For this review, take the finished solid that the model builds, in its own axes (mm). A direction names the side the tool comes from. Round coordinates to 2 decimals unless told otherwise and drop trailing zeros. Write each loop counter-clockwise with the first axis right and the second up, starting at its lowest first coordinate (ties: lowest second). Pieces come first, ordered by that corner, then holes.
from build123d import *

# Parameters (mm, degrees)
F0_W     = 20
F0_H     = 23
F0_R     = 2
F1_DEPTH = 3
F2_W     = 20
F2_H     = 3
F3_DEPTH = 20
F4_R     = 2
F5_DEPTH = 3.001
F7_DEPTH = 2
F9_DEPTH = 2
F10_SIZE = 1


with BuildPart() as f1:
    # F0 (on Top) → F1 (new body)
    with BuildSketch(Plane.XY):
        with Locations((10, -11.5)):
            Rectangle(F0_W, F0_H)
        with Locations((10, -13)):
            Circle(F0_R, mode=Mode.SUBTRACT)
    extrude(amount=F1_DEPTH)

    # F2 (on face) → F3 (join)
    with BuildSketch(Plane.XY.offset(3)):
        with Locations((10, -1.5)):
            Rectangle(F2_W, F2_H)
    extrude(amount=F3_DEPTH)

    # F4 (on face) → F5 (cut, through all)
    with BuildSketch(Plane.XZ.offset(3)):
        with Locations((10, 13)):
            Circle(F4_R)
    extrude(amount=-F5_DEPTH, mode=Mode.SUBTRACT)

    # F6 (on face) → F7 (join)
    with BuildSketch(Plane.YZ.offset(20)):
        Polygon((-3, 3), (-3, 23), (-23, 3), align=None)
    extrude(amount=-F7_DEPTH)

    # F8 (on face) → F9 (join)
    with BuildSketch(Plane(origin=(0, 0, 0), x_dir=(0, -1, 0), z_dir=(-1, 0, 0))):
        Polygon((23, 3), (3, 23), (3, 3), align=None)
    extrude(amount=-F9_DEPTH)

    # F10
    f10_edges = [f1.edges().sort_by_distance(p)[0] for p in [
        (8, -13, 3),
        (8, -3, 13),
    ]]
    chamfer(f10_edges, length=F10_SIZE)


solid = f1.part
(1) For faces 1 (the face through (6, -13, 3)), 2 (the face through (10, -1, 23)), list the 3-axis set-ups (+Z, -Z, +X, -X, +Y, -Y) from which the entire face can be reached by the end or side of a thin tool; tool diameter is ignored.
Geometry check:
face 1: +Z, -Y
face 2: +Z, +X, -X, +Y, -Y
(2) We need section C-C, the plane z = 13. Give the boundary of the cut face in (x, y).
Geometry check:
outline: (0, -13) - (2, -13) - (2, -3) - (7, -3) - (8, -2) - (8, 0) - (0, 0) - close; (12, -2) - (13, -3) - (18, -3) - (18, -13) - (20, -13) - (20, 0) - (12, 0) - close
(3) We need section B-B, the plane y = -13. Give the boundary of the cut face in (x, z).
Geometry check:
outline: (0, 0) - (8, 0) - (8, 2) - (7, 3) - (2, 3) - (2, 13) - (0, 13) - close; (12, 0) - (20, 0) - (20, 13) - (18, 13) - (18, 3) - (13, 3) - (12, 2) - close
(4) We need section D-D, the plane z = 3.5. Give the boundary of the cut face in (x, y).
Geometry check:
outline: (0, -22.5) - (2, -22.5) - (2, -3) - (18, -3) - (18, -22.5) - (20, -22.5) - (20, 0) - (0, 0) - close
(5) For pin 1 Ø5 at (x, z) = (9, 6) entering from -Y; pin 2 Ø3 at (y, z) = (-10.5, 20) entering from -X, all flat-tipped, find the tip position at first contact; note any pin that passes through.
Geometry check:
pin 1: stops at y = -3
pin 2: passes through
(6) We need section A-A, the plane x = 10. Give the boundary of the cut face in (y, z), and give its area (3 significant figures).
Geometry check:
outline: (-23, 0) - (-15, 0) - (-15, 2) - (-16, 3) - (-23, 3) - close; (-11, 0) - (0, 0) - (0, 11) - (-2, 11) - (-3, 10) - (-3, 3) - (-10, 3) - (-11, 2) - close; (-3, 16) - (-2, 15) - (0, 15) - (0, 23) - (-3, 23) - close
area: 103 mm2
(7) Mouldability with a two-part tool opening along Y and no side actions: class faces 3 (the face through (19, -13, 13)), 4 (the face through (10, -11, 1)), 5 (the face through (20, -9, 9)) as pulls with the +Y half, pulls with the -Y half, needs draft (parallel to the pull), parting line crosses it, or undercut.
Geometry check:
face 3: pulls with the -Y half
face 4: undercut
face 5: needs draft
(8) For line 1 along X through (y, z) = (-15.75, 5.75); line 2 along Z through (x, y) = (10, -1.25); line 3 along Y through (x, z) = (7.5, 16), list the stretches that pass through material, from the lowest coordinate up.
Geometry check:
line 1: x = 0 to 2, 18 to 20
line 2: z = 0 to 11, 15 to 23
line 3: y = -3 to 0
